from build123d import *

# Parameters (mm, degrees)
BOSS_EXTRUDE1_DEPTH = 2.3
SKETCH3_W           = 8
SKETCH3_H           = 3
SKETCH3_W_2         = 23
SKETCH3_H_2         = 32
CUT_EXTRUDE1_DEPTH  = 3.3
SKETCH4_R           = 1
CUT_EXTRUDE2_DEPTH  = 3.3
SKETCH6_R           = 1.15
CUT_EXTRUDE3_DEPTH  = 3.3
SKETCH8_R           = 1
CUT_EXTRUDE4_DEPTH  = 3.3
SKETCH9_W           = 10
SKETCH9_H           = 2.3
CUT_EXTRUDE5_DEPTH  = 2.3
CUT_EXTRUDE6_DEPTH  = 2.3
FILLET1_R           = 2


with BuildPart() as part:
    # Sketch2 → Boss-Extrude1 (new body)
    with BuildSketch(Plane(origin=(0, 0, 0), x_dir=(1, 0, 0), z_dir=(0, 1, 0))):
        Polygon((0, 35), (-49.5, 35), (-49.5, 0), (-49.5, -50), (0, -50), (49.5, -50), (49.5, 0), (49.5, 35), align=None)
    extrude(amount=BOSS_EXTRUDE1_DEPTH)

    # Sketch3 → Cut-Extrude1 (cut, through all)
    with BuildSketch(Plane(origin=(0, 2.3, 0), x_dir=(1, 0, 0), z_dir=(0, 1, 0))):
        with Locations((-45.5, 33.5)):
            Rectangle(SKETCH3_W, SKETCH3_H)
        with Locations((45.5, 33.5)):
            Rectangle(SKETCH3_W, SKETCH3_H)
        with Locations((38, -15)):
            Rectangle(SKETCH3_W_2, SKETCH3_H_2)
        with Locations((-38, -15)):
            Rectangle(SKETCH3_W_2, SKETCH3_H_2)
    extrude(amount=-CUT_EXTRUDE1_DEPTH, mode=Mode.SUBTRACT)

    # Sketch4 → Cut-Extrude2 (cut, through all)
    with BuildSketch(Plane(origin=(0, 2.3, 0), x_dir=(1, 0, 0), z_dir=(0, 1, 0))):
        with Locations((-45.5, 24)):
            Circle(SKETCH4_R)
        with Locations((45.5, 24)):
            Circle(SKETCH4_R)
    extrude(amount=-CUT_EXTRUDE2_DEPTH, mode=Mode.SUBTRACT)

    # Sketch6 → Cut-Extrude3 (cut, through all)
    with BuildSketch(Plane(origin=(0, 2.3, 0), x_dir=(1, 0, 0), z_dir=(0, 1, 0))):
        with Locations((0, -15)):
            Circle(SKETCH6_R)
        with Locations((-18.75, -4.825)):
            Circle(SKETCH6_R)
        with Locations((-18.75, -25.175)):
            Circle(SKETCH6_R)
        with Locations((18.75, -4.825)):
            Circle(SKETCH6_R)
        with Locations((18.75, -25.175)):
            Circle(SKETCH6_R)
    extrude(amount=-CUT_EXTRUDE3_DEPTH, mode=Mode.SUBTRACT)

    # Sketch8 → Cut-Extrude4 (cut, through all)
    with BuildSketch(Plane(origin=(0, 2.3, 0), x_dir=(1, 0, 0), z_dir=(0, 1, 0))):
        with Locations((-35, 32)):
            Circle(SKETCH8_R)
        with Locations((35, 32)):
            Circle(SKETCH8_R)
    extrude(amount=-CUT_EXTRUDE4_DEPTH, mode=Mode.SUBTRACT)

    # Sketch9 → Cut-Extrude5 (cut)
    with BuildSketch(Plane(origin=(0, 2.3, 0), x_dir=(1, 0, 0), z_dir=(0, 1, 0))):
        with Locations((-15, -43.85)):
            Rectangle(SKETCH9_W, SKETCH9_H)
        with Locations((15, -43.85)):
            Rectangle(SKETCH9_W, SKETCH9_H)
    extrude(amount=-CUT_EXTRUDE5_DEPTH, mode=Mode.SUBTRACT)

    # Sketch10 → Cut-Extrude6 (cut)
    with BuildSketch(Plane(origin=(0, 2.3, 0), x_dir=(1, 0, 0), z_dir=(0, 1, 0))):
        Polygon((0, 8), (25, 8), (25, 23), (-25, 23), (-25, 8), align=None)
    extrude(amount=-CUT_EXTRUDE6_DEPTH, mode=Mode.SUBTRACT)

    # Fillet1
    fillet1_edges = [part.edges().sort_by_distance(p)[0] for p in [
        (-25, 1.15, -8),
        (-25, 1.15, -23),
        (25, 1.15, -23),
        (25, 1.15, -8),
    ]]
    fillet(fillet1_edges, radius=FILLET1_R)


solid = part.part
Model file for the job. Use its own axes, mm. A direction names the side the tool comes from. Give positions to 0.01 mm unless a question says otherwise; leave off trailing zeros. Order: outer loops, then holes, each group sorted by start corner. A loop starts at its lowest first (then second) coordinate and runs counter-clockwise, first axis right, second up. Notation, with made-up numbers: (84, 22.25) - (103, 22.25) arc R13 ccw to (103, 32.25) - close; hole circle Ø8 at (-39.75, 31.5). An arc over 180 degrees is marked (long way). One line per item, written item: value.
Item 1: Two-plate mould, pull along Z, no slides. Class faces 1 (the flat face through (-1, 1, 50)), 2 (the flat face through (-15, 1, 42.7)), 3 (the flat face through (1, 1, -35)): released by +Z, released by -Z, zero draft, split by the parting line, or undercut.
Response values:
face 1: released by +Z
face 2: undercut
face 3: released by -Z
Item 2: Slice it at B-B (z = 15). List the corners of the cut face in (x, y).
Response values:
outline: (-26.5, 0) - (-1.15, 0) - (-1.15, 2.3) - (-26.5, 2.3) - close; (1.15, 0) - (26.5, 0) - (26.5, 2.3) - (1.15, 2.3) - close
Item 3: Wall check: line 1 (X direction, y = 1.7, z = -24); line 2 (Z direction, x = 18.75, y = 1.3) (3 decimals); line 3 (Z direction, x = 14, y = 1.5). Give the ranges that are in metal, low to high.
Response values:
line 1: -49.5 to -46.5, -44.5 to 44.5, 46.5 to 49.5
line 2: -35 to -23, -8 to 3.675, 5.975 to 24.025, 26.325 to 42.7, 45 to 50
line 3: -35 to -23, -8 to 42.7, 45 to 50
Item 4: Pin check, flat tip, straight feed: pin 1 Ø1.2 at (x, z) = (35, -32) entering from +Y. Stop position of the tip, or through.
Response values:
pin 1: through
Item 5: Tool access for faces 4 (the flat face through (-46, 1, -32)), 5 (the flat face through (-1, 0, 7)), 6 (the flat face through (41.5, 1, -33)), 7 (the flat face through (-20, 1, 44)), 8 (the flat face through (26.5, 1, 15)): list every direction of +Z, -Z, +X, -X, +Y, -Y with a clear straight run to the whole face (end or side of a thin tool).
Response values:
face 4: -Z, -X, +Y, -Y
face 5: +Z, -Z, +X, -X, -Y
face 6: -Z, +X, +Y, -Y
face 7: +Y, -Y
face 8: +X, +Y, -Y
Item 6: Slice it at D-D (x = 0). List the corners of the cut face in (y, z).
Response values:
outline: (0, -35) - (2.3, -35) - (2.3, -23) - (0, -23) - close; (0, -8) - (2.3, -8) - (2.3, 13.85) - (0, 13.85) - close; (0, 16.15) - (2.3, 16.15) - (2.3, 50) - (0, 50) - close
Item 7: Slice it at A-A (x = -30). List the corners of the cut face in (y, z), then the cut area to 3 significant figures.
Response values:
outline: (0, -35) - (2.3, -35) - (2.3, -1) - (0, -1) - close; (0, 31) - (2.3, 31) - (2.3, 50) - (0, 50) - close
area: 122 mm2
Item 8: Slice it at C-C (x = 18.75). List the corners of the cut face in (y, z) (3 decimals), then the cut area to 3 significant figures.
Response values:
outline: (0, -35) - (2.3, -35) - (2.3, -23) - (0, -23) - close; (0, -8) - (2.3, -8) - (2.3, 3.675) - (0, 3.675) - close; (0, 5.975) - (2.3, 5.975) - (2.3, 24.025) - (0, 24.025) - close; (0, 26.325) - (2.3, 26.325) - (2.3, 42.7) - (0, 42.7) - close; (0, 45) - (2.3, 45) - (2.3, 50) - (0, 50) - close
area: 145 mm2
